Could you check a few things on this drawing? It's one solid part, dimensions in mm from its lowest x, y, z. Give positions to 0.01 mm unless a question says otherwise; leave off trailing zeros. Order: outer loops, then holes, each group sorted by start corner. A loop starts at its lowest first (then second) coordinate and runs counter-clockwise, first axis right, second up.
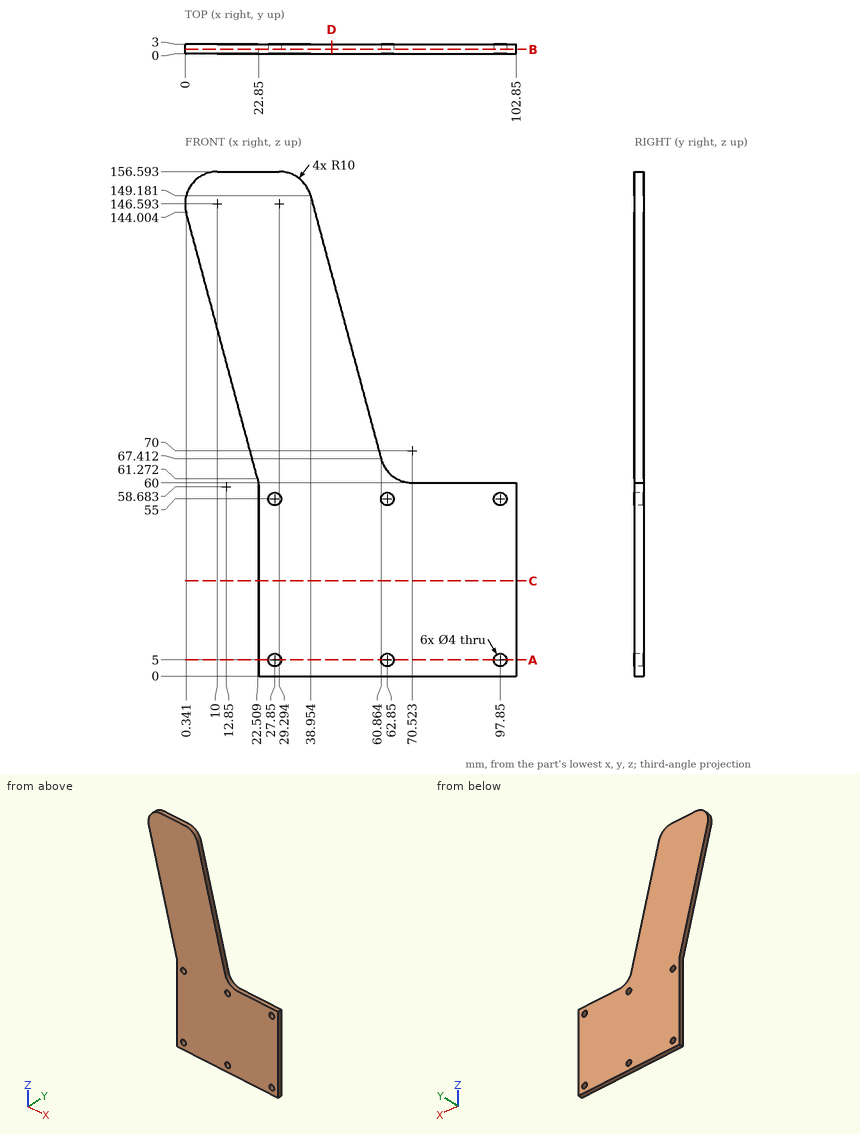
Q1. I'm going to push flat-ended pins straight in: P1, Ø1.5, axis at x = 47, z = 73, coming from the -Y side; P2, Ø0.9, axis at x = 79.5, y = 1, coming from the +Z side. Where does each tip first touch, or does it pass through?
Filled sheet:
P1: stops at y = 0
P2: stops at z = 60
Q2. I need wall thicknesses on L1, parallel to X at y = 2.3, z = 55; L2, parallel to Z at x = 98, y = 0.2 (1 decimal); L3, parallel to Z at x = 80, y = 0.65. Which ranges of each line are inside material? Lowest first, please.
Filled sheet:
L1: x = 22.85 to 25.85, 29.85 to 60.85, 64.85 to 95.85, 99.85 to 102.85
L2: z = 0 to 3, 7 to 53, 57 to 60
L3: z = 0 to 60
Q3. If we section it at C-C on z = 29.5: List the corners of the cut face in (x, y) for me, plus the area to 3 significant figures.
Filled sheet:
outline: (22.85, 0) - (102.85, 0) - (102.85, 3) - (22.85, 3) - close
area: 240 mm2
Q4. If we section it at D-D on x = 45.5: List the corners of the cut face in (y, z) for me.
Filled sheet:
outline: (0, 0) - (3, 0) - (3, 124.75) - (0, 124.75) - close
Q5. If we section it at A-A on z = 5: List the corners of the cut face in (x, y) for me, plus the area to 3 significant figures.
Filled sheet:
outline: (22.85, 0) - (25.85, 0) - (25.85, 3) - (22.85, 3) - close; (29.85, 0) - (60.85, 0) - (60.85, 3) - (29.85, 3) - close; (64.85, 0) - (95.85, 0) - (95.85, 3) - (64.85, 3) - close; (99.85, 0) - (102.85, 0) - (102.85, 3) - (99.85, 3) - close
area: 204 mm2
Q6. If we section it at B-B on y = 1.3: Give the number of separate pieces and of enclosed holes in the cut face, plus the area to 3 significant figures.
Filled sheet:
separate pieces: 1
enclosed holes: 6
area: 8,550 mm2
